Source: CAD feature listing. Evaluate the final solid. Frame: model axes, mm. Face numbers are marked on the shaded views. A direction names the side the tool comes from. Give positions to 0.01 mm unless a question says otherwise; leave off trailing zeros. Write each loop counter-clockwise with the first axis right and the second up, starting at its lowest first coordinate (ties: lowest second). Pieces come first, ordered by that corner, then holes. Notation, with made-up numbers: (87, 85) - (94, 85) arc R11 cw to (94, 99) - close; hole circle Ø8 at (27.25, 63.5). An arc over 180 degrees is marked (long way). One line per question, with ' | ' between items. Start each with the question number.
(1) Section A-A, the plane y = 80. State how many separate pieces and enclosed holes the cut face has, plus the area to 3 significant figures.
(2) Pin query (flat end, axial travel): pin 1 (1.2 mm diameter, centred on x = 178, z = -125.5, fed in from +Y); pin 2 (6 mm diameter, centred on x = 12, z = -126, fed in from +Y); pin 3 (1.3 mm diameter, centred on x = 164.46, z = -114.61, fed in from -Y); pin 4 (4 mm diameter, centred on x = 161, z = -18, fed in from +Y). Return the tip coordinate at first contact, or that it passes through.
(3) Ray query, line 1 (Z direction, x = 180, y = 93.5); line 2 (X direction, y = 34.5, z = -42); line 3 (Y direction, x = 85.5, z = -112.5). Return the intervals inside material, ascending. Write a range as [from, to].
(4) Section C-C, the plane z = -37. Return loops of the section in (x, y), plus the area to 3 significant figures.
(5) Access query for the marked faces 1 and 2. Directions: +Z, -Z, +X, -X, +Y, -Y. A direction counts if a zero-diameter tool reaches every point of the face in a straight line with its end or side. Return the directions, or none.
(6) Section B-B, the plane x = 122.5. Return loops of the section in (y, z).
(7) Draft query along X for the marked faces 3, 4 and 5. Return one class per face: +X half, -X half, draft (parallel to the pull), parting line (faces both ways), or undercut.
```python
from build123d import *
from build123d.topology import SkipClean

# Parameters (mm, degrees)
BOSS_EXTRUDE1_DEPTH     = 6.35
SKETCH2_W               = 203.2
SKETCH2_H               = 152.4
SKETCH2_R               = 1.1
SKETCH2_W_2             = 187.96
SKETCH2_H_2             = 137.16
BOSS_EXTRUDE2_DEPTH     = 101.6
SKETCH3_R               = 1.1
CUT_EXTRUDE1_DEPTH      = 12.7
CUT_EXTRUDE2_DEPTH      = 7.62
SKETCH6_R               = 11
CUT_EXTRUDE3_DEPTH      = 0.4
CUT_EXTRUDE6_DEPTH      = 3.25
SKETCH6_3_R             = 11
CUT_EXTRUDE16_DEPTH     = 2.12
CUT_EXTRUDE17_DEPTH     = 3.25
CUT_EXTRUDE18_DEPTH     = 0.5
SKETCH7_8_R             = 1.1
CUT_EXTRUDE10_DEPTH     = 3.175
CUT_EXTRUDE22_START     = -7.62
CUT_EXTRUDE22_DEPTH     = 7.62
CUT_EXTRUDE24_DEPTH     = 2.12
SKETCH20_W              = 0.4
SKETCH20_H              = 15.612494996
CUT_EXTRUDE26_DEPTH     = 3.25
CUT_EXTRUDE27_DEPTH     = 0.5
CUT_EXTRUDE28_DEPTH     = 3.25
SKETCH20_7_R            = 1.1
CUT_EXTRUDE29_DEPTH     = 3.175
SKETCH21_W              = 10
SKETCH21_H              = 20
CUT_EXTRUDE31_DEPTH     = 7.62
CUT_EXTRUDE32_START     = -6.35
CUT_EXTRUDE32_OUTLINE_R = 1.1
CUT_EXTRUDE32_DEPTH     = 3.175
CUT_EXTRUDE33_START     = -6.35
CUT_EXTRUDE33_OUTLINE_R = 1.1
CUT_EXTRUDE33_DEPTH     = 3.175
SKETCH20_9_R            = 1.1
CUT_EXTRUDE34_DEPTH     = 10.16


# Read off the part's stored shape, not the designer's step: Cut-Extrude32, Cut-Extrude33
with BuildPart() as part:
    # Sketch1 → Boss-Extrude1 (new body)
    with BuildSketch(Plane(origin=(0, 0, 0), x_dir=(1, 0, 0), z_dir=(0, 1, 0))):
        Polygon((0.000990329, 152.399052943), (0, 152.399052943), (0, 0), (203.2, 0), (203.2, 152.4), (0.000990329, 152.4), align=None)
    extrude(amount=BOSS_EXTRUDE1_DEPTH)

    # Sketch2 → Boss-Extrude2 (add)
    with BuildSketch(Plane(origin=(0, 6.35, 0), x_dir=(1, 0, 0), z_dir=(0, 1, 0))):
        with Locations((101.6, 76.2)):
            Rectangle(SKETCH2_W, SKETCH2_H)
        with Locations(Location((3.434665978, 148.463788162, 0), (0, 0, 270))):
            Circle(SKETCH2_R, mode=Mode.SUBTRACT)
        with Locations(Location((50.8, 148.463788162, 0), (0, 0, 270))):
            Circle(SKETCH2_R, mode=Mode.SUBTRACT)
        with Locations(Location((199.765334022, 148.463788162, 0), (0, 0, 270))):
            Circle(SKETCH2_R, mode=Mode.SUBTRACT)
        with Locations(Location((152.4, 148.463788162, 0), (0, 0, 270))):
            Circle(SKETCH2_R, mode=Mode.SUBTRACT)
        with Locations(Location((3.434665978, 3.936211838, 0), (0, 0, 270))):
            Circle(SKETCH2_R, mode=Mode.SUBTRACT)
        with Locations(Location((50.8, 3.936211838, 0), (0, 0, 270))):
            Circle(SKETCH2_R, mode=Mode.SUBTRACT)
        with Locations(Location((199.765334022, 3.936211838, 0), (0, 0, 270))):
            Circle(SKETCH2_R, mode=Mode.SUBTRACT)
        with Locations(Location((152.4, 3.936211838, 0), (0, 0, 270))):
            Circle(SKETCH2_R, mode=Mode.SUBTRACT)
        with Locations((101.6, 76.2)):
            Rectangle(SKETCH2_W_2, SKETCH2_H_2, mode=Mode.SUBTRACT)
    extrude(amount=BOSS_EXTRUDE2_DEPTH)

    # Sketch3 → Cut-Extrude1 (cut)
    with SkipClean():  # the faces are left unmerged after this step: merging them gives an invalid solid
        with BuildSketch(Plane.XZ):
            with Locations(Location((3.434665978, -3.936211838, 0), (0, 0, 270))):
                Circle(SKETCH3_R)
            with Locations(Location((50.8, -3.936211838, 0), (0, 0, 270))):
                Circle(SKETCH3_R)
            with Locations(Location((152.4, -3.936211838, 0), (0, 0, 270))):
                Circle(SKETCH3_R)
            with Locations(Location((199.765334022, -3.936211838, 0), (0, 0, 270))):
                Circle(SKETCH3_R)
            with Locations(Location((50.800247582, -148.463314633, 0), (0, 0, 270))):
                Circle(SKETCH3_R)
            with Locations(Location((3.434665978, -148.463314633, 0), (0, 0, 270))):
                Circle(SKETCH3_R)
            with Locations(Location((152.4, -148.463314633, 0), (0, 0, 270))):
                Circle(SKETCH3_R)
            with Locations(Location((199.765334022, -148.463314633, 0), (0, 0, 270))):
                Circle(SKETCH3_R)
        extrude(amount=-CUT_EXTRUDE1_DEPTH, mode=Mode.SUBTRACT)
    add(part.part.scale(1), mode=Mode.REPLACE)  # the faces are merged on a copy

    # Sketch5 → Cut-Extrude2 (cut)
    with BuildSketch(Plane(origin=(203.2, 0, 0), x_dir=(0, 0, -1), z_dir=(1, 0, 0))):
        with BuildLine():
            ThreePointArc((126.4, 7.09999974), (131.349747468, 9.150252272), (133.4, 14.09999974))
            Line((133.4, 14.09999974), (126.4, 14.09999974))
            Line((126.4, 14.09999974), (126.4, 7.09999974))
        make_face()
        with BuildLine():
            Line((126.4, 14.09999974), (133.4, 14.09999974))
            ThreePointArc((133.4, 14.09999974), (121.450252532, 19.049747208), (126.4, 7.09999974))
            Line((126.4, 7.09999974), (126.4, 14.09999974))
        make_face()
    extrude(amount=-CUT_EXTRUDE2_DEPTH, mode=Mode.SUBTRACT)

    # Sketch6 → Cut-Extrude3 (cut)
    with BuildSketch(Plane.ZY.offset(-195.58)):
        with Locations((-126.4, 14.09999974)):
            Circle(SKETCH6_R)
    extrude(amount=-CUT_EXTRUDE3_DEPTH, mode=Mode.SUBTRACT)

    # Sketch7 → Cut-Extrude6 (cut)
    with BuildSketch(Plane(origin=(0, 6.35, 0), x_dir=(1, 0, 0), z_dir=(0, 1, 0))):
        Polygon((176.812976287, 126.4), (176.812976287, 118.15), (179.312976287, 118.15), (179.312976287, 126.4), (179.312976287, 134.65), (176.812976287, 134.65), align=None)
    extrude(amount=-CUT_EXTRUDE6_DEPTH, mode=Mode.SUBTRACT)

    # Sketch6<3> → Cut-Extrude16 (cut)
    with BuildSketch(Plane.ZY.offset(-195.58)):
        with Locations((-126.4, 14.09999974)):
            Circle(SKETCH6_3_R)
    extrude(amount=-CUT_EXTRUDE16_DEPTH, mode=Mode.SUBTRACT)

    # Sketch7<9> → Cut-Extrude17 (cut)
    with BuildSketch(Plane(origin=(0, 6.35, 0), x_dir=(1, 0, 0), z_dir=(0, 1, 0))):
        Polygon((195.2, 118.593752244), (195.2, 126.4), (195.2, 134.206247756), (195.58, 134.206247756), (195.58, 118.593752244), align=None)
    extrude(amount=-CUT_EXTRUDE17_DEPTH, mode=Mode.SUBTRACT)

    # Sketch7<10> → Cut-Extrude18 (cut)
    with BuildSketch(Plane(origin=(0, 6.35, 0), x_dir=(1, 0, 0), z_dir=(0, 1, 0))):
        Polygon((179.312976287, 118.15), (195.2, 118.15), (195.2, 118.593752244), (195.2, 126.4), (195.2, 134.206247756), (195.2, 134.65), (179.312976287, 134.65), (179.312976287, 126.4), align=None)
    extrude(amount=-CUT_EXTRUDE18_DEPTH, mode=Mode.SUBTRACT)

    # Sketch7<8> → Cut-Extrude10 (cut)
    with BuildSketch(Plane(origin=(0, 6.35, 0), x_dir=(1, 0, 0), z_dir=(0, 1, 0))):
        with Locations(Location((187.256488143, 137.825, 0), (0, 0, 270))):
            Circle(SKETCH7_8_R)
        with Locations(Location((187.256488143, 114.975, 0), (0, 0, 270))):
            Circle(SKETCH7_8_R)
        with Locations(Location((164.462976287, 138.19, 0), (0, 0, 270))):
            Circle(SKETCH7_8_R)
        with Locations(Location((164.462976287, 114.61, 0), (0, 0, 270))):
            Circle(SKETCH7_8_R)
    extrude(amount=-CUT_EXTRUDE10_DEPTH, mode=Mode.SUBTRACT)

    # Sketch17 → Cut-Extrude22 (cut)
    with BuildSketch(Plane.ZY.offset(CUT_EXTRUDE22_START)):
        with BuildLine():
            ThreePointArc((-119.4, 14.1), (-126.4, 21.1), (-133.4, 14.1))
            Line((-133.4, 14.1), (-126.4, 14.1))
            Line((-126.4, 14.1), (-126.4, 7.1))
            ThreePointArc((-126.4, 7.1), (-121.450252532, 9.150252532), (-119.4, 14.1))
        make_face()
        with BuildLine():
            Line((-126.4, 14.1), (-133.4, 14.1))
            ThreePointArc((-133.4, 14.1), (-131.349747468, 9.150252532), (-126.4, 7.1))
            Line((-126.4, 7.1), (-126.4, 14.1))
        make_face()
    extrude(amount=CUT_EXTRUDE22_DEPTH, mode=Mode.SUBTRACT)

    # Sketch18 → Cut-Extrude24 (cut)
    # profile 1 of 2: a face of its own
    with BuildSketch(Plane(origin=(7.62, 0, 0), x_dir=(0, 0, -1), z_dir=(1, 0, 0))):
        with BuildLine():
            ThreePointArc((134.206247498, 6.35), (136.570268494, 9.908861878), (137.4, 14.1))
            ThreePointArc((137.4, 14.1), (122.208861878, 24.270268494), (118.593752502, 6.35))
            Line((118.593752502, 6.35), (134.206247498, 6.35))
        make_face()
        with BuildLine():
            ThreePointArc((133.4, 14.1), (131.349747468, 9.150252532), (126.4, 7.1))
            ThreePointArc((126.4, 7.1), (119.4, 14.1), (126.4, 21.1))
            ThreePointArc((126.4, 21.1), (131.349747468, 19.049747468), (133.4, 14.1))
        make_face(mode=Mode.SUBTRACT)
    # profile 2 of 2: a face of its own
    with BuildSketch(Plane(origin=(7.62, 0, 0), x_dir=(0, 0, -1), z_dir=(1, 0, 0))):
        with BuildLine():
            Line((134.206247498, 6.35), (118.593752502, 6.35))
            ThreePointArc((118.593752502, 6.35), (126.4, 3.1), (134.206247498, 6.35))
        make_face()
    extrude(amount=-CUT_EXTRUDE24_DEPTH, mode=Mode.SUBTRACT)

    # Sketch20 → Cut-Extrude26 (cut)
    with BuildSketch(Plane(origin=(0, 6.35, 0), x_dir=(1, 0, 0), z_dir=(0, 1, 0))):
        with Locations((7.82, 126.4)):
            Rectangle(SKETCH20_W, SKETCH20_H)
    extrude(amount=-CUT_EXTRUDE26_DEPTH, mode=Mode.SUBTRACT)

    # Sketch20<4> → Cut-Extrude27 (cut)
    with BuildSketch(Plane(origin=(0, 6.35, 0), x_dir=(1, 0, 0), z_dir=(0, 1, 0))):
        Polygon((8.02, 118.15), (8.02, 118.593752502), (8.02, 134.206247498), (8.02, 134.65), (19.92, 134.65), (19.92, 126.4), (19.92, 118.15), align=None)
    extrude(amount=-CUT_EXTRUDE27_DEPTH, mode=Mode.SUBTRACT)

    # Sketch20<5> → Cut-Extrude28 (cut)
    with BuildSketch(Plane(origin=(0, 6.35, 0), x_dir=(1, 0, 0), z_dir=(0, 1, 0))):
        Polygon((19.92, 118.15), (22.42, 118.15), (22.42, 126.4), (22.42, 134.65), (19.92, 134.65), (19.92, 126.4), align=None)
    extrude(amount=-CUT_EXTRUDE28_DEPTH, mode=Mode.SUBTRACT)

    # Sketch20<7> → Cut-Extrude29 (cut)
    with BuildSketch(Plane(origin=(0, 6.35, 0), x_dir=(1, 0, 0), z_dir=(0, 1, 0))):
        with Locations(Location((13.97, 137.825, 0), (0, 0, 270))):
            Circle(SKETCH20_7_R)
        with Locations(Location((13.97, 114.975, 0), (0, 0, 270))):
            Circle(SKETCH20_7_R)
        with Locations(Location((34.77, 138.825, 0), (0, 0, 270))):
            Circle(SKETCH20_7_R)
    extrude(amount=-CUT_EXTRUDE29_DEPTH, mode=Mode.SUBTRACT)

    # Sketch21 → Cut-Extrude31 (cut)
    with BuildSketch(Plane.XY):
        with Locations((96.6, 97.95)):
            Rectangle(SKETCH21_W, SKETCH21_H)
        Polygon((111.6, 107.95), (101.6, 107.95), (101.6, 87.95), (111.6, 87.95), (111.6, 88.914389003), align=None)
    extrude(amount=-CUT_EXTRUDE31_DEPTH, mode=Mode.SUBTRACT)

    # Cut-Extrude32 outline → Cut-Extrude32 (cut)
    with BuildSketch(Plane(origin=(0, 6.35, 0), x_dir=(1, 0, 0), z_dir=(0, 1, 0)).offset(CUT_EXTRUDE32_START)):
        with Locations((13.97, 137.825)):
            Circle(CUT_EXTRUDE32_OUTLINE_R)
        with Locations((34.77, 138.825)):
            Circle(CUT_EXTRUDE32_OUTLINE_R)
        with Locations((13.97, 114.975)):
            Circle(CUT_EXTRUDE32_OUTLINE_R)
    extrude(amount=CUT_EXTRUDE32_DEPTH, mode=Mode.SUBTRACT)

    # Cut-Extrude33 outline → Cut-Extrude33 (cut)
    with BuildSketch(Plane(origin=(0, 6.35, 0), x_dir=(1, 0, 0), z_dir=(0, 1, 0)).offset(CUT_EXTRUDE33_START)):
        with Locations((164.462976287, 138.19)):
            Circle(CUT_EXTRUDE33_OUTLINE_R)
        with Locations((164.462976287, 114.61)):
            Circle(CUT_EXTRUDE33_OUTLINE_R)
        with Locations((187.256488143, 114.975)):
            Circle(CUT_EXTRUDE33_OUTLINE_R)
        with Locations((187.256488143, 137.825)):
            Circle(CUT_EXTRUDE33_OUTLINE_R)
    extrude(amount=CUT_EXTRUDE33_DEPTH, mode=Mode.SUBTRACT)

    # Sketch20<9> → Cut-Extrude34 (cut)
    with BuildSketch(Plane(origin=(0, 6.35, 0), x_dir=(1, 0, 0), z_dir=(0, 1, 0))):
        with Locations(Location((34.77, 113.975, 0), (0, 0, 270))):
            Circle(SKETCH20_9_R)
    extrude(amount=-CUT_EXTRUDE34_DEPTH, mode=Mode.SUBTRACT)


solid = part.part
```
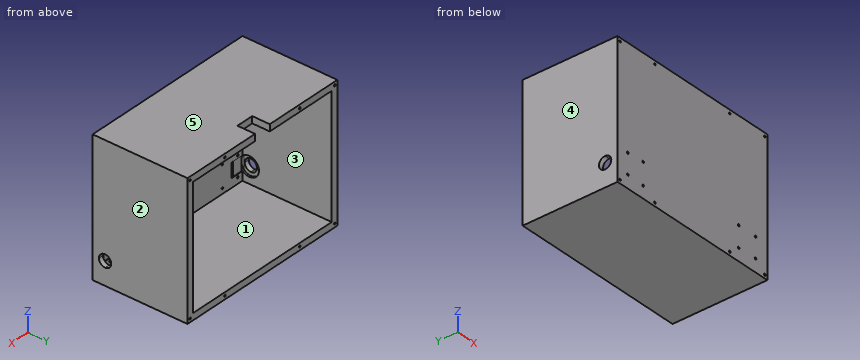
Check sheet entries:
1) separate pieces: 1 | enclosed holes: 9 | area: 5,160 mm²
2) pin 1: y = 3.1 | pin 2: y = 5.85 | pin 3: through | pin 4: y = 6.35
3) line 1: [-152.4, -144.78], [-7.62, 0] | line 2: [0, 7.62], [195.58, 203.2] | line 3: [0, 6.35]
4) outline: (0, 0) - (203.2, 0) - (203.2, 107.95) - (195.58, 107.95) - (195.58, 6.35) - (7.62, 6.35) - (7.62, 107.95) - (0, 107.95) - close | area: 2,840 mm²
5) face 1: +Y | face 2: +Z, -Z, +X, +Y, -Y
6) outline: (0, -152.4) - (107.95, -152.4) - (107.95, -144.78) - (6.35, -144.78) - (6.35, -7.62) - (107.95, -7.62) - (107.95, 0) - (0, 0) - close
7) face 3: undercut | face 4: -X half | face 5: draft
